The listing builds one solid part. Answer for the finished solid, in the listing's coordinates (mm). A direction names the side the tool comes from. Give positions to 0.01 mm unless a question says otherwise; leave off trailing zeros. Write each loop counter-clockwise with the first axis right and the second up, starting at its lowest first coordinate (ties: lowest second). Pieces come first, ordered by that corner, then holes.
```python
from build123d import *

# Parameters (mm, degrees)
SKETCH1_W           = 22.75
SKETCH1_H           = 12.5
BOSS_EXTRUDE1_DEPTH = 22.5
BOSS_EXTRUDE2_DEPTH = 4.4
SKETCH3_R           = 2.365
BOSS_EXTRUDE3_DEPTH = 3.25
SKETCH4_W           = 12.5
SKETCH4_H           = 2.5
BOSS_EXTRUDE4_DEPTH = 5
SKETCH5_W           = 12.5
SKETCH5_H           = 2.5
BOSS_EXTRUDE5_DEPTH = 5
CUT_EXTRUDE1_DEPTH  = 36.487673916
FILLET1_R           = 0.5


with BuildPart() as part:
    # Sketch1 → Boss-Extrude1 (new body)
    with BuildSketch(Plane(origin=(0, 0, 0), x_dir=(1, 0, 0), z_dir=(0, 1, 0))):
        with Locations((11.375, -6.25)):
            Rectangle(SKETCH1_W, SKETCH1_H)
    extrude(amount=BOSS_EXTRUDE1_DEPTH)

    # Sketch2 → Boss-Extrude2 (add)
    with BuildSketch(Plane(origin=(0, 22.5, 0), x_dir=(1, 0, 0), z_dir=(0, 1, 0))):
        with BuildLine():
            ThreePointArc((11.812373594, -3.4), (0, -6.25), (11.812373594, -9.1))
            ThreePointArc((11.812373594, -9.1), (14.662373594, -6.25), (11.812373594, -3.4))
        make_face()
    extrude(amount=BOSS_EXTRUDE2_DEPTH)

    # Sketch3 → Boss-Extrude3 (add)
    with BuildSketch(Plane(origin=(0, 26.9, 0), x_dir=(1, 0, 0), z_dir=(0, 1, 0))):
        with Locations(Location((6.25, -6.25, 0), (0, 0, 90))):
            Circle(SKETCH3_R)
    extrude(amount=BOSS_EXTRUDE3_DEPTH)

    # Sketch4 → Boss-Extrude4 (add)
    with BuildSketch(Plane(origin=(22.75, 0, 0), x_dir=(0, 0, -1), z_dir=(1, 0, 0))):
        with Locations((-6.25, 17)):
            Rectangle(SKETCH4_W, SKETCH4_H)
    extrude(amount=BOSS_EXTRUDE4_DEPTH)

    # Sketch5 → Boss-Extrude5 (add)
    with BuildSketch(Plane.ZY):
        with Locations((6.25, 17)):
            Rectangle(SKETCH5_W, SKETCH5_H)
    extrude(amount=BOSS_EXTRUDE5_DEPTH)

    # Sketch6 → Cut-Extrude1 (cut, through all)
    with BuildSketch(Plane(origin=(0, 18.25, 0), x_dir=(1, 0, 0), z_dir=(0, 1, 0))):
        with BuildLine():
            Line((27.75, -5.65), (27.75, -6.85))
            Line((27.75, -6.85), (26.55, -6.85))
            ThreePointArc((26.55, -6.85), (24.75, -6.25), (26.55, -5.65))
            Line((26.55, -5.65), (27.75, -5.65))
        make_face()
        with BuildLine():
            Line((-5, -6.85), (-5, -5.65))
            Line((-5, -5.65), (-3.8, -5.65))
            ThreePointArc((-3.8, -5.65), (-2, -6.25), (-3.8, -6.85))
            Line((-3.8, -6.85), (-5, -6.85))
        make_face()
    extrude(amount=-CUT_EXTRUDE1_DEPTH, mode=Mode.SUBTRACT)

    # Fillet1
    fillet1_edges = [part.edges().sort_by_distance(p)[0] for p in [
        (22.75, 7.875, 0),
        (22.75, 7.875, 12.5),
        (0, 7.875, 0),
        (0, 7.875, 12.5),
        (0, 20.375, 0),
        (22.75, 20.375, 0),
        (22.75, 20.375, 12.5),
        (0, 20.375, 12.5),
    ]]
    fillet(fillet1_edges, radius=FILLET1_R)


solid = part.part
```
Item 1: Consider probe 1 along Z at (x, y) = (-3, 17); probe 2 along X at (y, z) = (15, 6.25); probe 3 along Y at (x, z) = (26.5, 3.25). Determine where each line is inside the solid, lowest interval first.
Conclusion:
probe 1: z = 0 to 5.25, 7.25 to 12.5
probe 2: x = 0 to 22.75
probe 3: y = 15.75 to 18.25
Item 2: A cutting plane is placed at D-D, the plane x = 21. Give the vertices of the cut face in (y, z).
Conclusion:
outline: (0, 0) - (22.5, 0) - (22.5, 12.5) - (0, 12.5) - close
Item 3: Which of the six approach directions +Z, -Z, +X, -X, +Y, -Y give full straight-line access (tool end or side, diameter ignored) to faces 1 (the face through (9, 26.9, 6)), 2 (the face through (0, 8, 6)), 3 (the face through (14.66, 24.67, 6.31))?
Conclusion:
face 1: +Y
face 2: +Z, -Z, -X, -Y
face 3: +X, +Y
Item 4: A cutting plane is placed at C-C, the plane z = 4.75. Give the vertices of the cut face in (x, y).
Conclusion:
outline: (-5, 15.75) - (0, 15.75) - (0, 0) - (22.75, 0) - (22.75, 15.75) - (27.75, 15.75) - (27.75, 18.25) - (22.75, 18.25) - (22.75, 22.5) - (14.24, 22.5) - (14.24, 26.9) - (8.08, 26.9) - (8.08, 30.15) - (4.42, 30.15) - (4.42, 26.9) - (0.18, 26.9) - (0.18, 22.5) - (0, 22.5) - (0, 18.25) - (-5, 18.25) - close
Item 5: A cutting plane is placed at A-A, the plane x = -3. Give the vertices of the cut face in (y, z).
Conclusion:
outline: (15.75, 0) - (18.25, 0) - (18.25, 5.25) - (15.75, 5.25) - close; (15.75, 7.25) - (18.25, 7.25) - (18.25, 12.5) - (15.75, 12.5) - close
Item 6: A cutting plane is placed at B-B, the plane y = 21. Give the vertices of the cut face in (x, z), plus the area to 3 significant figures.
Conclusion:
outline: (0, 0.5) arc R0.5 ccw to (0.5, 0) - (22.25, 0) arc R0.5 ccw to (22.75, 0.5) - (22.75, 12) arc R0.5 ccw to (22.25, 12.5) - (0.5, 12.5) arc R0.5 ccw to (0, 12) - close
area: 284 mm2
Item 7: Each of these flat-tipped pins is pushed along its axis until it touches: P1, Ø5, axis at x = 2, z = 3, coming from the +Y side; P2, Ø1.6, axis at x = 24, z = 5.5, coming from the -Y side; P3, Ø6, axis at y = 5.5, z = 7.5, coming from the +X side. Where does it stop, or does it pass through?
Conclusion:
P1: stops at y = 26.9
P2: stops at y = 15.75
P3: stops at x = 22.75
